Can you work these out from the model? Positions are in its coordinate system, mm. Give positions to 0.01 mm unless a question says otherwise; leave off trailing zeros. Loops run counter-clockwise (first coordinate to the right, second up) from the corner with the lowest first, then second, coordinate; pieces in that order, holes last. Notation, with made-up numbers: M 88,39.5 L 114,39.5 A14 ccw 114,44.5 Z; hole C 60.25,87.5 d11. An arc over 180 degrees is marked long. Use CSV: the item, a comma, the result in double quotes.
from build123d import *

# Parameters (mm, degrees)
FILLET2_R = 2
FILLET3_R = 0.5


with BuildPart() as part:
    # Sketch1 → Revolve1 (revolve)
    with BuildSketch(Plane.XY, mode=Mode.PRIVATE) as revolve1_sk:
        Polygon((25.5, 0), (23.5, 0), (23.5, -2), (27.5, -2), (27.5, 5.5), (25.5, 5.5), (24.5, 3.5), (25.5, 3.5), align=None)
    revolve(revolve1_sk.sketch.rotate(Axis((0, 0, 0), (0, 1, 0)), 90), axis=Axis((0, 0, 0), (0, 1, 0)))

    # Fillet2
    fillet2_edges = [part.edges().sort_by_distance(p)[0] for p in [
        (0, -2, 27.5),
        (0, 5.5, 27.5),
    ]]
    fillet(fillet2_edges, radius=FILLET2_R - 0.0001)  # a hair under: the kernel refuses the full size

    # Fillet3
    fillet3_edges = [part.edges().sort_by_distance(p)[0] for p in [
        (0, -2, 23.5),
    ]]
    fillet(fillet3_edges, radius=FILLET3_R)


solid = part.part
Q1. If we mould it in two halves opening along Z, with no side actions, what happens to faces 1 (the cylindrical face through (24.397, 1.775, -12.69)), 2 (the cylindrical face through (-23.3, -0.76, 3.06)), 3 (the flat face through (15, -2, 19))? For each: released by +Z, released by -Z, zero draft, split by the parting line, or undercut.
Model answer:
face 1,"split by the parting line"
face 2,"undercut"
face 3,"zero draft"
Q2. I want a section at C-C, the plane y = 1.5. Please give me the cut outline in (x, z), then the cut area to 3 significant figures.
Model answer:
outline,"C 0,0 d55; hole C 0,0 d51"
area,"333 mm2"
Q3. Please list where these lines run through material, in increasing order: L1, parallel to X at y = 2.15, z = 0; L2, parallel to X at y = 1.75, z = 12; L3, parallel to Z at x = -2.5, y = 2.5. Write a range as from..to.
Model answer:
L1,"-27.5..-25.5, 25.5..27.5"
L2,"-24.74..-22.5, 22.5..24.74"
L3,"-27.39..-25.38, 25.38..27.39"
Q4. I'm going to push flat-ended pins straight in: P1, Ø12, axis at x = 9.5, z = -13, coming from the +Y side; P2, Ø3, axis at x = 16.5, y = 2, coming from the +Z side. Where does each tip first touch, or does it pass through?
Model answer:
P1,"through"
P2,"z = 23.05"
